Design review of the part shown in the three views and the two pictorial views. Dimensions are in mm from the part's minimum x, y and z. Give positions to 0.01 mm unless a question says otherwise; leave off trailing zeros. Loops run counter-clockwise (first coordinate to the right, second up) from the corner with the lowest first, then second, coordinate; pieces in that order, holes last. Notation, with made-up numbers: (-2.75, -35.5) - (6.25, -35.5) arc R34 cw to (6.25, -3.5) - close; hole circle Ø9 at (-18, -28.75). An arc over 180 degrees is marked (long way). Answer in a Markdown table with one row per item.
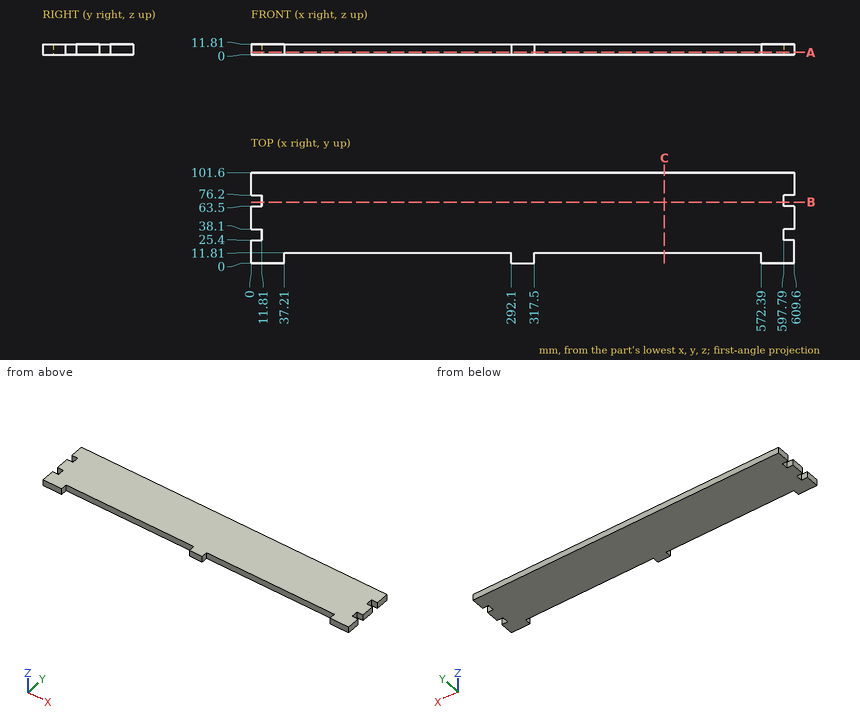
1. Clearance check with flat-ended pins moving along their axes: pin 1 (1 mm diameter, centred on y = 70.5, z = 8.5, fed in from +X); pin 2 (3.5 mm diameter, centred on x = 402.5, z = 7.5, fed in from -Y); pin 3 (1 mm diameter, centred on y = 36, z = 6.5, fed in from -X). State where each tip first meets the part, or that it passes through.
Values:
| item | result |
|---|---|
| pin 1 | stops at x = 597.79 |
| pin 2 | stops at y = 11.81 |
| pin 3 | stops at x = 11.81 |
2. We need section C-C, the plane x = 463.5. Give the boundary of the cut face in (y, z), and give its area (3 significant figures).
Values:
| item | result |
|---|---|
| outline | (11.81, 0) - (101.6, 0) - (101.6, 11.81) - (11.81, 11.81) - close |
| area | 1,060 mm^2 |
3. We need section B-B, the plane y = 68.5. Give the boundary of the cut face in (x, z).
Values:
| item | result |
|---|---|
| outline | (11.81, 0) - (597.79, 0) - (597.79, 11.81) - (11.81, 11.81) - close |
4. Wall thickness on line 1 (X direction, y = 8.5, z = 7.5); line 2 (X direction, y = 70, z = 3.25); line 3 (Y direction, x = 563.5, z = 10): over which ranges is each line inside the solid? List them lowest first. Write a range as [from, to].
Values:
| item | result |
|---|---|
| line 1 | x = [0, 37.21], [292.1, 317.5], [572.39, 609.6] |
| line 2 | x = [11.81, 597.79] |
| line 3 | y = [11.81, 101.6] |
5. We need section A-A, the plane z = 2.5. Give the boundary of the cut face in (x, y).
Values:
| item | result |
|---|---|
| outline | (0, 0) - (37.21, 0) - (37.21, 11.81) - (292.1, 11.81) - (292.1, 0) - (317.5, 0) - (317.5, 11.81) - (572.39, 11.81) - (572.39, 0) - (609.6, 0) - (609.6, 25.4) - (597.79, 25.4) - (597.79, 38.1) - (609.6, 38.1) - (609.6, 63.5) - (597.79, 63.5) - (597.79, 76.2) - (609.6, 76.2) - (609.6, 101.6) - (0, 101.6) - (0, 76.2) - (11.81, 76.2) - (11.81, 63.5) - (0, 63.5) - (0, 38.1) - (11.81, 38.1) - (11.81, 25.4) - (0, 25.4) - close |
